Could you check a few things on this model? Use its own coordinates, in mm. A direction names the side the tool comes from. Give positions to 0.01 mm unless a question says otherwise; leave off trailing zeros. Order: outer loops, then holes, each group sorted by start corner. A loop starts at its lowest first (then second) coordinate and runs counter-clockwise, first axis right, second up.
(1) Imagine slicing it at A-A, the plane x = -191. Write out the boundary of the cut face in (y, z), then the cut area to 3 significant figures.
(2) Will these pins go through, and if not, where does the flat tip stop? pin 1 (4 mm diameter, centred on x = -290, y = 0, fed in from -Z); pin 2 (5 mm diameter, centred on y = -4, z = -9.5, fed in from -X); pin 3 (4 mm diameter, centred on x = -212, y = 4, fed in from +Z).
(3) If we mould it in two halves opening along X, with no side actions, what happens to faces 1 (the flat face through (2, -1, 2)), 2 (the flat face through (3.72, 0.06, -25.56)), 3 (the flat face through (-36.305, -4.493, 3.288))? For each: released by +X, released by -X, zero draft, split by the parting line, or undercut.
(4) If I drill on probe 1 along X at (y, z) = (0, -20.45); probe 2 along Y at (x, z) = (-205, -21.5); probe 3 along X at (y, z) = (0, -26.75), over which ranges is the centre line in solid material (lowest first)?
(5) On a 3-axis mill with a long thin cutter (end or side, diameter ignored), from which of +Z, -Z, +X, -X, +Y, -Y can I reach the whole of each face in a straight line? I mean faces 4 (the flat face through (-203, 0, -18.641)), 5 (the flat face through (-120, 5, -32)), 6 (the cylindrical face through (-0.9, 2.04, 4.05)). Say none if no direction works.
(6) Imagine slicing it at B-B, the plane x = -59. Write out the boundary of the cut face in (y, z).
from build123d import *

# Parameters (mm, degrees)
BOSS_EXTRUDE1_DEPTH       = 5
M5X0_8_TAPPED_HOLE1_D     = 4.2
SKETCH5_R                 = 4.15
CUT_EXTRUDE1_DEPTH        = 6
M4X0_7_TAPPED_HOLE1_D     = 3.3
M4X0_7_TAPPED_HOLE1_DEPTH = 15
M4X0_7_TAPPED_HOLE1_TIP   = 0.991420021
FILLET1_R                 = 2.5
CHAMFER1_SIZE             = 1
F_1_0MM_DOWEL_HOLE1_D     = 1
F_1_0MM_DOWEL_HOLE1_DEPTH = 5
F_1_0MM_DOWEL_HOLE1_TIP   = 0.30043031


with BuildPart() as part:
    # Sketch2 → Boss-Extrude1 (new body, symmetric)
    with BuildSketch(Plane(origin=(0, 0, 0), x_dir=(1, 0, 0), z_dir=(0, 1, 0))):
        with BuildLine():
            Line((-210, 50.641016151), (-20, 50.641016151))
            ThreePointArc((-20, 50.641016151), (-12, 48.497422612), (-6.143593539, 42.641016151))
            Line((-6.143593539, 42.641016151), (13.856406461, 8))
            ThreePointArc((13.856406461, 8), (12.25671109, -10.284601755), (-5.472322293, -15.035081933))
            Line((-5.472322293, -15.035081933), (-70, 8.451072039))
            Line((-70, 8.451072039), (-70, 18.641016151))
            Line((-70, 18.641016151), (-340, 18.641016151))
            Line((-340, 18.641016151), (-340, 33.641016151))
            Line((-340, 33.641016151), (-210, 50.641016151))
        make_face()
    extrude(amount=BOSS_EXTRUDE1_DEPTH, both=True)

    # M5x0.8 Tapped Hole1 (through all)
    with Locations(Plane(origin=(0, 5, 0), x_dir=(1, 0, 0), z_dir=(0, 1, 0))):
        with Locations((-20, 34.641016151), (0, 0)):
            Hole(M5X0_8_TAPPED_HOLE1_D / 2)

    # Sketch5 → Cut-Extrude1 (cut)
    with BuildSketch(Plane(origin=(0, 5, 0), x_dir=(1, 0, 0), z_dir=(0, 1, 0))):
        Circle(SKETCH5_R)
    extrude(amount=-CUT_EXTRUDE1_DEPTH, mode=Mode.SUBTRACT)

    # M4x0.7 Tapped Hole1
    with Locations(Plane.XY.offset(-18.641016151)):
        with Locations((-290, 0), (-120, 0)):
            Hole(M4X0_7_TAPPED_HOLE1_D / 2, depth=M4X0_7_TAPPED_HOLE1_DEPTH)
            with Locations((0, 0, -(M4X0_7_TAPPED_HOLE1_DEPTH + M4X0_7_TAPPED_HOLE1_TIP / 2))):  # 118° drill point
                Cone(0, M4X0_7_TAPPED_HOLE1_D / 2, M4X0_7_TAPPED_HOLE1_TIP, mode=Mode.SUBTRACT)

    # Fillet1
    fillet1_edges = [part.edges().sort_by_distance(p)[0] for p in [
        (-70, 0, -8.451072039),
        (-340, 0, -33.641016151),
        (-210, 0, -50.641016151),
    ]]
    fillet(fillet1_edges, radius=FILLET1_R)

    # Chamfer1
    chamfer1_edges = [part.edges().sort_by_distance(p)[0] for p in [
        (-70, -5, -14.421303518),
        (-205, -5, -18.641016151),
        (-114.918615686, -5, -50.641016151),
        (-12, -5, -48.497422612),
        (-205, 5, -18.641016151),
        (-70, 5, -14.421303518),
        (12.25671109, 5, 10.284601755),
        (3.856406461, 5, -25.320508076),
        (-12, 5, -48.497422612),
        (-273.992778821, -5, -42.27272969),
        (-273.992778821, 5, -42.27272969),
        (-36.913686326, -5, 3.5913613),
        (-340, -5, -25.043835126),
        (-69.547880111, -5, -8.767649794),
        (-339.37888369, -5, -33.095834527),
        (-209.999656106, -5, -50.635734213),
        (-340, 5, -25.043835126),
        (-36.913686326, 5, 3.5913613),
        (-69.547880111, 5, -8.767649794),
        (-339.37888369, 5, -33.095834527),
        (-209.999656106, 5, -50.635734213),
        (-114.918615686, 5, -50.641016151),
        (3.856406461, -5, -25.320508076),
        (12.25671109, -5, 10.284601755),
    ]]
    chamfer(chamfer1_edges, length=CHAMFER1_SIZE)

    # Ø1.0mm Dowel Hole1
    with Locations(Plane.XY.offset(-18.641016151)):
        with Locations((-205, 0)):
            Hole(F_1_0MM_DOWEL_HOLE1_D / 2, depth=F_1_0MM_DOWEL_HOLE1_DEPTH)
            with Locations((0, 0, -(F_1_0MM_DOWEL_HOLE1_DEPTH + F_1_0MM_DOWEL_HOLE1_TIP / 2))):  # 118° drill point
                Cone(0, F_1_0MM_DOWEL_HOLE1_D / 2, F_1_0MM_DOWEL_HOLE1_TIP, mode=Mode.SUBTRACT)


solid = part.part
Answer block:
1. outline: (-5, -49.64) - (-4, -50.64) - (4, -50.64) - (5, -49.64) - (5, -19.64) - (4, -18.64) - (-4, -18.64) - (-5, -19.64) - close
1. area: 318 mm2
2. pin 1: stops at z = -40.44
2. pin 2: stops at x = -70
2. pin 3: stops at z = -18.64
3. face 1: undercut
3. face 2: released by +X
3. face 3: released by -X
4. probe 1: x = -340 to -291.65, -288.35 to -205.5, -204.5 to -121.65, -118.35 to 6.67
4. probe 2: y = -5 to -0.5, 0.5 to 5
4. probe 3: x = -340 to -291.65, -288.35 to -121.65, -118.35 to 3.03
5. face 4: +Z, -X, +Y, -Y
5. face 5: +Z, -Z, +X, -X, +Y
5. face 6: +Y
6. outline: (-5, -49.64) - (-4, -50.64) - (4, -50.64) - (5, -49.64) - (5, -5.51) - (4, -4.45) - (-4, -4.45) - (-5, -5.51) - close
